Can you work these out from the model? Positions are in its coordinate system, mm. A direction names the side the tool comes from. Coordinates: 2 decimals unless noted, no trailing zeros. Loops run counter-clockwise (first coordinate to the right, second up) from the corner with the lowest first, then second, coordinate; pieces in that order, holes last.
Autodesk Inventor part; units mm, degrees
ref_plane "YZ Plane" through (0, 0, 0) normal (1, 0, 0) x (0, 1, 0)
ref_plane "XZ Plane" through (0, 0, 0) normal (0, 1, 0) x (-1, 0, 0)
ref_plane "XY Plane" through (0, 0, 0) normal (0, 0, 1) x (1, 0, 0)
sketch "スケッチ1" plane through (0, 0, 0) normal (1, 0, 0) x (0, 1, 0)
  line L0 (7, 0) -> (7, 0)
  line L1 (0, -9) -> (0, -14)
  line L2 (0, -14) -> (27, -14)
  line L3 (27, -14) -> (27, -11)
  line L4 (27, -11) -> (25, -11)
  line L5 (25, -11) -> (25, 0)
  line L6 (25, 0) -> (7, 0)
  line L7 (7, 0) -> (4.1, 0)
  line L8 (4.1, 0) -> (4.1, -9)
  line L9 (4.1, -9) -> (0, -9)
  point P0 (0, 0)
  dimension "d2" = 11
  dimension "d3" = 3
  dimension "d4" = 25
  dimension "d5" = 2
  dimension "d35" = 0
  dimension "d36" = 7
  dimension "d37" = 4.1
  dimension "d45" = 9
revolve "回転1" add sketch "スケッチ1" angle 360 about axis through (0, 0, -9) along (0, 0, -1)
chamfer "面取り1" distance 1 angle 45 1 edges at (0, -25, 0)
sketch "スケッチ2" plane through (0, 0, -14) normal (0, 0, -1) x (-1, 0, 0)
  point P0 (0, 0)
hole "穴1" at (0, 0, -14) direction (0, 0, 1) diameter 4.3 end through all
sketch "スケッチ3" plane through (0, 0, -14) normal (0, 0, -1) x (-1, 0, 0)
  circle A0 centre (0, 0) radius 21
  point P0 (0, 0)
  point P1 (0, -21)
  point P2 (18.1865, -10.5)
  point P3 (18.1865, 10.5)
  point P4 (0, 21)
  point P5 (-18.1865, 10.5)
  point P6 (-18.1865, -10.5)
  dimension "d20" = 42
  dimension "d23" = 360
hole "穴2" at (0, -21, -14) at (-18.1865, -10.5, -14) at (-18.1865, 10.5, -14) at (0, 21, -14) at (18.1865, 10.5, -14) at (18.1865, -10.5, -14) direction (0, 0, 1) diameter 3.2 end through all
chamfer "面取り4" distance 0.5 angle 45 1 edges at (0, -4.1, 0)
properties part number "base3" material "ABS プラスチック"
Item 1: We'd pull the mould along Y, two halves only. Please class faces 1 (the face through (-0.09, -2.15, -11.46)), 2 (the face through (18.12, -12.1, -6.9)), 3 (the face through (26.36, -5.85, -12.48)), 4 (the face through (0, 5, 0)): +Y half, -Y half, draft (parallel to the pull), parting line (faces both ways), or undercut.
Results are:
face 1: undercut
face 2: undercut
face 3: parting line
face 4: draft
Item 2: Suppose I cut it at B-B, the plane y = 0. Please give me the cut outline in (x, z), plus the area to 3 significant figures.
Results are:
outline: (-27, -14) - (-2.15, -14) - (-2.15, -9) - (-4.1, -9) - (-4.1, -0.5) - (-4.6, 0) - (-24, 0) - (-25, -1) - (-25, -11) - (-27, -11) - close; (2.15, -14) - (27, -14) - (27, -11) - (25, -11) - (25, -1) - (24, 0) - (4.6, 0) - (4.1, -0.5) - (4.1, -9) - (2.15, -9) - close
area: 615 mm2
Item 3: On a 3-axis mill with a long thin cutter (end or side, diameter ignored), from which of +Z, -Z, +X, -X, +Y, -Y can I reach the whole of each face in a straight line? I mean faces 5 (the face through (-1.08, 19.82, -6.9)), 6 (the face through (-2, 2, -9)). Say none if no direction works.
Results are:
face 5: +Z, -Z
face 6: +Z
Item 4: Suppose I cut it at A-A, the plane x = 0. Please give me the cut outline in (y, z), plus the area to 3 significant figures.
Results are:
outline: (-27, -14) - (-22.6, -14) - (-22.6, 0) - (-24, 0) - (-25, -1) - (-25, -11) - (-27, -11) - close; (-19.4, -14) - (-2.15, -14) - (-2.15, -9) - (-4.1, -9) - (-4.1, -0.5) - (-4.6, 0) - (-19.4, 0) - close; (2.15, -14) - (19.4, -14) - (19.4, 0) - (4.6, 0) - (4.1, -0.5) - (4.1, -9) - (2.15, -9) - close; (22.6, -14) - (27, -14) - (27, -11) - (25, -11) - (25, -1) - (24, 0) - (22.6, 0) - close
area: 526 mm2
Item 5: I'm going to push flat-ended pins straight in: P1, Ø1.9, axis at x = -18.19, y = 10.5, coming from the -Z side; P2, Ø1.5, axis at y = -20.5, z = -5.5, coming from the -X side; P3, Ø5.5, axis at x = 0, y = 0, coming from the +Z side; P4, Ø6, axis at x = 0.5, z = -6, coming from the +Y side. Where does each tip first touch, or does it pass through?
Results are:
P1: passes through
P2: stops at x = -15.33
P3: stops at z = -9
P4: stops at y = 25
Item 6: Suppose I cut it at D-D, the plane z = -5.5. Please give me the cut outline in (x, y).
Results are:
outline: circle Ø50 at (0, 0); hole circle Ø3.2 at (-18.19, -10.5); hole circle Ø3.2 at (-18.19, 10.5); hole circle Ø8.2 at (0, 0); hole circle Ø3.2 at (0, -21); hole circle Ø3.2 at (0, 21); hole circle Ø3.2 at (18.19, -10.5); hole circle Ø3.2 at (18.19, 10.5)
Item 7: Suppose I cut it at C-C, the plane z = -12.5. Please give me the cut outline in (x, y).
Results are:
outline: circle Ø54 at (0, 0); hole circle Ø3.2 at (-18.19, -10.5); hole circle Ø3.2 at (-18.19, 10.5); hole circle Ø4.3 at (0, 0); hole circle Ø3.2 at (0, -21); hole circle Ø3.2 at (0, 21); hole circle Ø3.2 at (18.19, -10.5); hole circle Ø3.2 at (18.19, 10.5)
Item 8: I need wall thicknesses on line 1 along X through (y, z) = (-10.5, -2.75); line 2 along X through (y, z) = (0, -12.4); line 3 along Y through (x, z) = (1, -0.25). Which ranges of each line are inside material? Lowest first, please.
Results are:
line 1: x = -22.69 to -19.79, -16.59 to 16.59, 19.79 to 22.69
line 2: x = -27 to -2.15, 2.15 to 27
line 3: y = -24.23 to -22.25, -19.75 to -4.23, 4.23 to 19.75, 22.25 to 24.23
